Autodesk Inventor part; units mm, degrees
ref_plane "YZ Plane" through (0, 0, 0) normal (1, 0, 0) x (0, 1, 0)
ref_plane "XZ Plane" through (0, 0, 0) normal (0, 1, 0) x (-1, 0, 0)
ref_plane "XY Plane" through (0, 0, 0) normal (0, 0, 1) x (1, 0, 0)
sketch "Sketch1" plane through (0, 0, 0) normal (0, 1, 0) x (-1, 0, 0)
  line L0 (0, -63.5) -> (38.1, -63.5)
  line L1 (38.1, -63.5) -> (38.1, 0)
  line L2 (38.1, 0) -> (0, 0)
  line L3 (0, 0) -> (0, -63.5)
  line L4 (28.575, -31.75) -> (28.575, -50.8)
  line L5 (22.225, -50.8) -> (22.225, -31.75)
  arc A0 (28.575, -31.75) -> (22.225, -31.75) centre (25.4, -31.75) ccw
  arc A1 (22.225, -50.8) -> (28.575, -50.8) centre (25.4, -50.8) ccw
  circle A2 centre (12.7, -15.875) radius 3.175
  dimension "d0" = 38.1
  dimension "d2" = 63.5
  dimension "d3" = 19.05
  dimension "d4" = 50.8
  dimension "d5" = 12.7
  dimension "d6" = 15.875
  dimension "d7" = 25.4
  dimension "d10" = 3.175
  dimension "d11" = 3.175
  dimension "d12" = 6.35
extrude "Extrusion1" add sketch "Sketch1" along normal blind 3.175
equation "\"d2\" = 1.66667 * d0"
equation "\"d3\" = 0.5 * d0"
equation "\"d4\" = 0.8 * d2"
equation "\"d5\" = 0.333333 * d0"
equation "\"d6\" = 0.25 * d2"
equation "\"d7\" = 0.666667 * d0"
equation "\"d10\" = d8"
equation "\"d11\" = d8"
equation "\"d12\" = 2 * d8"
equation "\"d8\" = 0.05 * d2"
properties part number "8.2 Q1"
Geometry: final body of the model. Coordinates: model frame, mm. A direction names the side the tool comes from. Coordinates: 2 decimals unless noted, no trailing zeros. Order: outer loops, then holes, each group sorted by start corner. A loop starts at its lowest first (then second) coordinate and runs counter-clockwise, first axis right, second up. Notation, with made-up numbers: (4.25, 48.5) -> (57.25, 48.5) arc R35 cw to (57.25, 86.5) -> close; hole circle Ø5 at (-20.5, 84.5). An arc over 180 degrees is marked (long way). Write each question's results on one line, items separated by ' | '. Start each with the question number.
1) Material intervals for line 1 along Z through (x, y) = (-12.7, 0.7); line 2 along X through (y, z) = (2.15, -38) (3 decimals); line 3 along X through (y, z) = (1.25, -18.5), sorted ascending.
2) Set-up query: faces 5 (the flat face through (-19, 2, -63.5)), 6 (the flat face through (-28.575, 2, -41)). Return all of +Z, -Z, +X, -X, +Y, -Y with unobstructed straight access to the full face (end or side cutting, diameter ignored); none if empty.
3) Cut plane B-B, the plane y = 0.85. Output: boundary loops of the cut face in (x, z) (3 decimals), and give its area (3 significant figures).
4) Cut plane C-C, the plane z = -17. Output: boundary loops of the cut face in (x, y) (3 decimals), and give its area (3 significant figures).
5) Cut plane A-A, the plane x = -12.7. Output: boundary loops of the cut face in (y, z) (3 decimals).
6) Mould query, pull axis X, two halves, no side actions, for faces 1 (the cylindrical face through (-9.528, 1.565, -16.015)), 2 (the cylindrical face through (-25.47, 1.565, -53.974)), 3 (the flat face through (0, 2, -31)), 4 (the flat face through (-19, 0, -31)). Classes: released by +X, released by -X, zero draft, split by the parting line, or undercut.
Checks:
1) line 1: -63.5 to -19.05, -12.7 to 0 | line 2: -38.1 to -28.575, -22.225 to 0 | line 3: -38.1 to -14.49, -10.91 to 0
2) face 5: -Z, +X, -X, +Y, -Y | face 6: +Y, -Y
3) outline: (-38.1, -63.5) -> (0, -63.5) -> (0, 0) -> (-38.1, 0) -> close; hole (-28.575, -50.8) arc R3.175 ccw to (-22.225, -50.8) -> (-22.225, -31.75) arc R3.175 ccw to (-28.575, -31.75) -> close; hole circle Ø6.35 at (-12.7, -15.875) | area: 2,240 mm^2
4) outline: (-38.1, 0) -> (-15.669, 0) -> (-15.669, 3.175) -> (-38.1, 3.175) -> close; (-9.731, 0) -> (0, 0) -> (0, 3.175) -> (-9.731, 3.175) -> close | area: 102 mm^2
5) outline: (0, -63.5) -> (3.175, -63.5) -> (3.175, -19.05) -> (0, -19.05) -> close; (0, -12.7) -> (3.175, -12.7) -> (3.175, 0) -> (0, 0) -> close
6) face 1: undercut | face 2: undercut | face 3: released by +X | face 4: zero draft
